Read the model definition and answer for the solid it produces. Units are mm, in the model's axes. A direction names the side the tool comes from. Coordinates: 2 decimals unless noted, no trailing zeros. Loops run counter-clockwise (first coordinate to the right, second up) from the corner with the lowest first, then second, coordinate; pieces in that order, holes last. Notation, with made-up numbers: (50, -27.75) - (103, -27.75) arc R30 cw to (103, 2.25) - close; hole circle Ø11 at (78, -13.75). An arc over 180 degrees is marked (long way). One line per item, written item: value. Start each with the question number.
from build123d import *

# Parameters (mm, degrees)
SKETCH1_W           = 80
SKETCH1_H           = 198
BOSS_EXTRUDE1_DEPTH = 5
SKETCH2_R           = 3.75
BOSS_EXTRUDE2_DEPTH = 7.5
CUT_EXTRUDE1_DEPTH  = 88.5
FILLET2_R           = 2


with BuildPart() as part:
    # Sketch1 → Boss-Extrude1 (new body)
    with BuildSketch(Plane(origin=(0, 0, 0), x_dir=(1, 0, 0), z_dir=(0, 1, 0))):
        Rectangle(SKETCH1_W, SKETCH1_H)
    extrude(amount=BOSS_EXTRUDE1_DEPTH)

    # Sketch2 → Boss-Extrude2 (add)
    with BuildSketch(Plane.ZY.offset(40)):
        with Locations((-64.928905814, 3.75)):
            Circle(SKETCH2_R)
        with Locations((59.5, 3.75)):
            Circle(SKETCH2_R)
    boss_extrude2 = extrude(amount=BOSS_EXTRUDE2_DEPTH)

    # Mirror1: Boss-Extrude2 across plane
    add(boss_extrude2.mirror(Plane(origin=(0, 0, 0), x_dir=(0, 0, 1), z_dir=(1, 0, 0))))

    # Sketch3 → Cut-Extrude1 (cut, through all)
    with BuildSketch(Plane.ZY.offset(40)):
        Polygon((-99, 5), (-72.932513489, -1.759148434), (-103.799311702, -1.759148434), align=None)
    extrude(amount=-CUT_EXTRUDE1_DEPTH, mode=Mode.SUBTRACT)

    # Fillet2
    fillet2_edges = [part.edges().sort_by_distance(p)[0] for p in [
        (40, 2.5, -89.358442796),
        (-40, 2.5, -89.358442796),
    ]]
    fillet(fillet2_edges, radius=FILLET2_R)


solid = part.part
1) Section A-A, the plane x = -2 is taken. Determine the outline of the cut face in (y, z), and give its area (3 significant figures).
2) Flat-ended cylindrical pins translate along their axes: P1, Ø10, axis at x = 22.5, z = -10, coming from the +Y side; P2, Ø4, axis at y = 3, z = 84.5, coming from the -X side; P3, Ø8, axis at x = -27.5, z = -29.5, coming from the -Y side; P4, Ø2.5, axis at y = 1.5, z = 76, coming from the +X side. Find the tip coordinate at first contact, or state that the pin passes through.
3) Straight lines are drawn through the part: L1, parallel to Y at x = 34, z = 54; L2, parallel to X at y = 0.5, z = 72; L3, parallel to Z at x = 43, y = 6.5. For each, find the intervals that lie inside material, in ascending order.
4) For faces 1 (the cylindrical face through (43.698, 4.876, 63.077)), 2 (the cylindrical face through (-43.698, 4.876, 63.077)), 3 (the flat face through (-47.5, 4, -65)), determine the directions among +Z, -Z, +X, -X, +Y, -Y from which every point of the face is accessible in a straight line to the end or side of a thin tool.
5) Section B-B, the plane z = 52 is taken. Determine the outline of the cut face in (x, y).
6) Determine the mould class of faces 4 (the flat face through (-1, 5, -1)), 5 (the flat face through (-1, 2, 99)), 6 (the flat face through (40, 2, -2)) for opening direction Z: released by +Z, released by -Z, zero draft, split by the parting line, or undercut.
Answer below:
1. outline: (0, -79.72) - (5, -99) - (5, 99) - (0, 99) - close
1. area: 942 mm2
2. P1: y = 5
2. P2: x = -40
2. P3: y = 0
2. P4: x = 40
3. L1: 0 to 5
3. L2: -40 to 40
3. L3: -67.48 to -62.38, 56.95 to 62.05
4. face 1: +X
4. face 2: -X
4. face 3: +Z, -Z, -X, +Y, -Y
5. outline: (-40, 0) - (40, 0) - (40, 5) - (-40, 5) - close
6. face 4: zero draft
6. face 5: released by +Z
6. face 6: undercut
